Here's how the part is built. I have some questions about the finished solid (model axes, mm). Face numbers are marked on the shaded views. A direction names the side the tool comes from. Coordinates: 2 decimals unless noted, no trailing zeros. Write each loop counter-clockwise with the first axis right and the second up, starting at its lowest first coordinate (ties: lowest second). Pieces come first, ordered by that corner, then holes.
Item 1: If we section it at B-B (z = 54): Please give me the cut outline in (x, y), then the cut area to 3 significant figures.
Item 2: If we section it at A-A (x = 90): Please give me the cut outline in (y, z).
Item 3: We'd pull the mould along Y, two halves only. Please class the marked faces 4, 5 and 6: +Y half, -Y half, draft (parallel to the pull), parting line (faces both ways), or undercut.
Item 4: For the marked faces 1, 2 and 3, which set-ups out of +Z, -Z, +X, -X, +Y, -Y let a thin tool reach every point of the face, with its end or its side?
Item 5: If we section it at C-C (z = 74): Please give me the cut outline in (x, y), then the cut area to 3 significant figures.
Item 6: If we section it at D-D (y = 52.5): Please give me the cut outline in (x, z).
Item 7: If I drill on line 1 (Z direction, x = 90, y = 41); line 2 (X direction, y = 95.25, z = 54); line 3 (Y direction, x = 90, z = 59), over which ranges is the centre line in solid material (lowest first)?
Item 8: I'm going to push flat-ended pins straight in: pin 1 Ø1.5 at (x, z) = (95.5, 68) entering from -Y; pin 2 Ø3.5 at (x, z) = (90, 54) entering from +Y; pin 3 Ø6 at (x, z) = (92.5, 37.5) entering from -Y; pin 4 Ø8 at (y, z) = (83.5, 54) entering from +X. Where does each tip first touch, or does it pass through?
from build123d import *

# Parameters (mm, degrees)
SKETCH005_AS_DRAWN_R                                = 2.75
EXTRUDE_SKETCH005001_DEPTH                          = 90
EXTRUDE_SKETCH005001_ONTO_SKETCH005_ROLL_ANGLE      = 90
EXTRUDE_SKETCH005001_ONTO_SKETCH005_PLACEMENT_ANGLE = 180
CYLINDER_R                                          = 9
CYLINDER_DEPTH                                      = 80
CYLINDER001_R                                       = 9
CYLINDER001_DEPTH                                   = 80
CYLINDER001_ROLL_ANGLE                              = 90


with BuildPart() as clone_of_sketch005_extrude001:
    # Sketch005 as drawn → Extrude_Sketch005001 (new)
    with BuildSketch(Plane.XY):
        with Locations((-90, 54)):
            Circle(SKETCH005_AS_DRAWN_R)
    extrude(amount=-EXTRUDE_SKETCH005001_DEPTH)


with BuildPart() as clone_of_sketch005_extrude001_1:
    # Extrude_Sketch005001 onto Sketch005 roll: moved
    add(clone_of_sketch005_extrude001.part.rotate(Axis((0, 0, 0), (1, 0, 0)), EXTRUDE_SKETCH005001_ONTO_SKETCH005_ROLL_ANGLE))


with BuildPart() as clone_of_sketch005_extrude001_2:
    # Extrude_Sketch005001 onto Sketch005 placement: moved
    add(clone_of_sketch005_extrude001_1.part.moved(Location((0, 111, 0))).rotate(Axis((0, 111, 0), (0, 0, 1)), EXTRUDE_SKETCH005001_ONTO_SKETCH005_PLACEMENT_ANGLE))


with BuildPart() as cilindro:
    # Cylinder → Cylinder (new body)
    with BuildSketch(Plane(origin=(76.968275, 45, 32), x_dir=(1, 0, 0), z_dir=(0, 0, 1))):
        Circle(CYLINDER_R)
    extrude(amount=CYLINDER_DEPTH)


with BuildPart() as clone_of_cilindro:
    # Clone003 base: copy of Cilindro
    add(cilindro.part)


with BuildPart() as clone_of_cilindro_1:
    # Clone003 placement: moved
    add(clone_of_cilindro.part.moved(Location((0, 50, 0))))


with BuildPart() as cut003:
    # Cylinder001 → Cylinder001 (new body)
    with BuildSketch(Plane.XY):
        Circle(CYLINDER001_R)
    extrude(amount=CYLINDER001_DEPTH)


with BuildPart() as cut003_1:
    # Cylinder001 roll: moved
    add(cut003.part.rotate(Axis((0, 0, 0), (1, 0, 0)), CYLINDER001_ROLL_ANGLE))


with BuildPart() as cut003_2:
    # Cylinder001 placement: moved
    add(cut003_1.part.moved(Location((76.9683, 110, 112))))

    # Fusion: union Clone of Cilindro, Cilindro
    add(clone_of_cilindro_1.part)
    add(cilindro.part)


with BuildPart() as cut003_3:
    # Fusion placement: moved
    add(cut003_2.part.moved(Location((13.0317, 0, -18))))

    # Cut003: cut Clone of Sketch005_Extrude001
    add(clone_of_sketch005_extrude001_2.part, mode=Mode.SUBTRACT)


solid = cut003_3.part
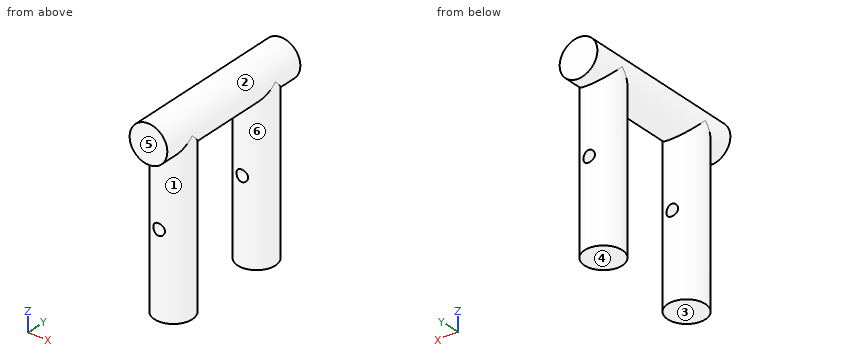
Answer list:
1. outline: (87.25, 36.43) - (87.25, 53.57) arc R9 ccw to start; (87.25, 86.43) - (87.25, 103.57) arc R9 ccw to start; (92.75, 36.43) arc R9 ccw to (92.75, 53.57) - close; (92.75, 86.43) arc R9 ccw to (92.75, 103.57) - close
1. area: 314 mm2
2. outline: (30, 85) - (36, 85) - (36, 56.75) - (54, 56.75) - (54, 85) - (86, 85) - (86, 56.75) - (104, 56.75) - (104, 85) - (110, 85) - (110, 103) - (30, 103) - close; (36, 14) - (54, 14) - (54, 51.25) - (36, 51.25) - close; (86, 14) - (104, 14) - (104, 51.25) - (86, 51.25) - close
3. face 4: draft
3. face 5: -Y half
3. face 6: undercut
4. face 1: -Z
4. face 2: none
4. face 3: -Z, +X, -X, +Y, -Y
5. outline: circle Ø18 at (90, 45); circle Ø18 at (90, 95)
5. area: 509 mm2
6. outline: (85.03, 14) - (94.97, 14) - (94.97, 86.5) arc R9 ccw (long way) to (85.03, 86.5) - close; hole circle Ø5.5 at (90, 54)
7. line 1: z = 14 to 51.25, 56.75 to 103
7. line 2: x = 81 to 87.25, 92.75 to 99
7. line 3: y = 36 to 54, 86 to 104
8. pin 1: stops at y = 37.36
8. pin 2: passes through
8. pin 3: stops at y = 36
8. pin 4: stops at x = 94.97
